The listing builds one solid part. Answer for the finished solid, in the listing's coordinates (mm). A direction names the side the tool comes from. Give positions to 0.01 mm unless a question says otherwise; leave off trailing zeros. Loops run counter-clockwise (first coordinate to the right, second up) from the corner with the lowest first, then second, coordinate; pieces in that order, holes last. Notation, with made-up numbers: (-2, -23.5) - (40, -23.5) arc R10 cw to (40, -16.5) - close; hole circle Ø11 at (7, 24). An arc over 180 degrees is marked (long way). Write item = value, one per line. Start each with the question number.
1) Flat-ended cylindrical pins translate along their axes: P1, Ø4, axis at y = 0, z = 0, coming from the +X side; P2, Ø3, axis at x = 6.5, y = -3.5, coming from the +Z side. Find the tip coordinate at first contact, or state that the pin passes through.
2) The part is cut by section A-A on z = 0. Write down the section's boundary in (x, y).
3) Which of the six approach directions +Z, -Z, +X, -X, +Y, -Y give full straight-line access (tool end or side, diameter ignored) to faces 5 (the cylindrical face through (8.004, -1.172, 8.923)), 6 (the cylindrical face through (4, -6, 0))?
4) Consider probe 1 along Z at (x, y) = (6.5, 0); probe 2 along X at (y, z) = (5, -5); probe 3 along Y at (x, z) = (3.25, 1). Determine where each line is inside the solid, lowest interval first.
5) The part is cut by section C-C on x = 4.75. Write down the section's boundary in (y, z).
6) The mould has two halves that part along X. Classify faces 1 (the flat face through (8.5, 2, -2)), 2 (the cylindrical face through (0.504, -1.172, 8.923)), 3 (the flat face through (0, -2, -2)), 4 (the flat face through (1, -2, -6)): +X half, -X half, draft (parallel to the pull), parting line (faces both ways), or undercut.
from build123d import *

# Parameters (mm, degrees)
SMUSSO1_SIZE = 0.25


with BuildPart() as part:
    # Schizzo1 → Rivoluzione1 (revolve)
    with BuildSketch(Plane.XY):
        Polygon((0, 2.5), (0, 9), (1, 9), (1, 6), (7.5, 6), (7.5, 9), (8.5, 9), (8.5, 2.5), align=None)
    revolve(axis=Axis((0, 0, 0), (1, 0, 0)))

    # Smusso1
    smusso1_edges = [part.edges().sort_by_distance(p)[0] for p in [
        (8.5, -9, 0),
        (7.5, -9, 0),
        (1, -9, 0),
        (0, -9, 0),
    ]]
    chamfer(smusso1_edges, length=SMUSSO1_SIZE)


solid = part.part
Answer below:
q1.P1 = through
q1.P2 = 8.59
q2.outline = (0, -8.75) - (0.25, -9) - (0.75, -9) - (1, -8.75) - (1, -6) - (7.5, -6) - (7.5, -8.75) - (7.75, -9) - (8.25, -9) - (8.5, -8.75) - (8.5, -2.5) - (0, -2.5) - close; (0, 2.5) - (8.5, 2.5) - (8.5, 8.75) - (8.25, 9) - (7.75, 9) - (7.5, 8.75) - (7.5, 6) - (1, 6) - (1, 8.75) - (0.75, 9) - (0.25, 9) - (0, 8.75) - close
q3.face_5 = +X, -X
q3.face_6 = none
q4.probe_1 = -6 to -2.5, 2.5 to 6
q4.probe_2 = 0 to 1, 7.5 to 8.5
q4.probe_3 = -5.92 to -2.29, 2.29 to 5.92
q5.outline = circle Ø12 at (0, 0); hole circle Ø5 at (0, 0)
q6.face_1 = +X half
q6.face_2 = draft
q6.face_3 = -X half
q6.face_4 = undercut
